Build history of the part. All positions in model axes, mm. A direction names the side the tool comes from. Give positions to 0.01 mm unless a question says otherwise; leave off trailing zeros. Order: outer loops, then holes, each group sorted by start corner. A loop starts at its lowest first (then second) coordinate and runs counter-clockwise, first axis right, second up. Notation, with made-up numbers: (-14, 76) - (-8, 76) arc R14 cw to (-8, 93) - close; hole circle Ø11 at (50.25, 83). An arc over 180 degrees is marked (long way). Use a Markdown table: item, result.
from build123d import *

# Parameters (mm, degrees)
F0_R     = 12.15
F1_DEPTH = 4.45


with BuildPart() as f1:
    # F0 (on Top) → F1 (new body)
    with BuildSketch(Plane.XY):
        Polygon((-46.197247, 20.387878), (-50.585262, 20.387878), (-50.585262, -13.197176), (-46.197247, -13.197176), (-46.197247, -30.152489), (25.432527, -30.152489), (29.882527, -30.152489), (29.882527, -13.418792), (25.432527, -13.418792), (25.432527, 20.387878), (29.882527, 20.387878), (29.882527, 37.746087), (25.432527, 37.746087), (-46.197247, 37.746087), align=None)
        with Locations((-10.38236, 3.484543)):
            Circle(F0_R, mode=Mode.SUBTRACT)
    extrude(amount=F1_DEPTH)


solid = f1.part
1) Wall check: line 1 (X direction, y = 3, z = 2); line 2 (X direction, y = 22.5, z = 0.95); line 3 (X direction, y = 14, z = 1.7). Give the ranges that are in metal, low to high. Write a range as from..to.
Computed:
| item | result |
|---|---|
| line 1 | x = -50.59..-22.52, 1.76..25.43 |
| line 2 | x = -46.2..29.88 |
| line 3 | x = -50.59..-16.47, -4.3..25.43 |
2) Slice it at D-D (y = -22.5). Write the cut outline in (x, z), and give its area (3 significant figures).
Computed:
| item | result |
|---|---|
| outline | (-46.2, 0) - (29.88, 0) - (29.88, 4.45) - (-46.2, 4.45) - close |
| area | 339 mm² |
3) Slice it at C-C (z = 3.35). Write the cut outline in (x, y), and give its area (3 significant figures).
Computed:
| item | result |
|---|---|
| outline | (-50.59, -13.2) - (-46.2, -13.2) - (-46.2, -30.15) - (29.88, -30.15) - (29.88, -13.42) - (25.43, -13.42) - (25.43, 20.39) - (29.88, 20.39) - (29.88, 37.75) - (-46.2, 37.75) - (-46.2, 20.39) - (-50.59, 20.39) - close; hole circle Ø24.3 at (-10.38, 3.48) |
| area | 4,700 mm² |
4) Pin check, flat tips, straight feed: P1, Ø1.3, axis at x = -47.5, z = 3, coming from the -Y side; P2, Ø2, axis at y = -22, z = 2, coming from the -X side; P3, Ø1.3, axis at x = -47.5, z = 2.5, coming from the +Y side. Stop position of each tip, or through.
Computed:
| item | result |
|---|---|
| P1 | stops at y = -13.2 |
| P2 | stops at x = -46.2 |
| P3 | stops at y = 20.39 |
5) Two-plate mould, pull along X, no slides. Class faces 1 (the flat face through (25.433, 3, 2)), 2 (the cylindrical face through (-4.776, -7.295, 2.194)), 3 (the flat face through (-48, 20.388, 2)), 4 (the flat face through (-50.585, 4, 2)): +X half, -X half, draft (parallel to the pull), parting line (faces both ways), or undercut.
Computed:
| item | result |
|---|---|
| face 1 | +X half |
| face 2 | undercut |
| face 3 | draft |
| face 4 | -X half |
6) Tool access for faces 5 (the flat face through (-46.197, 29, 2)), 6 (the flat face through (28, 20.388, 2)), 7 (the flat face through (-46.197, -22, 2)): list every direction of +Z, -Z, +X, -X, +Y, -Y with a clear straight run to the whole face (end or side of a thin tool).
Computed:
| item | result |
|---|---|
| face 5 | +Z, -Z, -X, +Y |
| face 6 | +Z, -Z, +X |
| face 7 | +Z, -Z, -X, -Y |
7) Slice it at B-B (x = -11). Write the cut outline in (y, z).
Computed:
| item | result |
|---|---|
| outline | (-30.15, 0) - (-8.65, 0) - (-8.65, 4.45) - (-30.15, 4.45) - close; (15.62, 0) - (37.75, 0) - (37.75, 4.45) - (15.62, 4.45) - close |
8) Slice it at A-A (y = -6). Write the cut outline in (x, z), and give its area (3 significant figures).
Computed:
| item | result |
|---|---|
| outline | (-50.59, 0) - (-17.98, 0) - (-17.98, 4.45) - (-50.59, 4.45) - close; (-2.79, 0) - (25.43, 0) - (25.43, 4.45) - (-2.79, 4.45) - close |
| area | 271 mm² |
